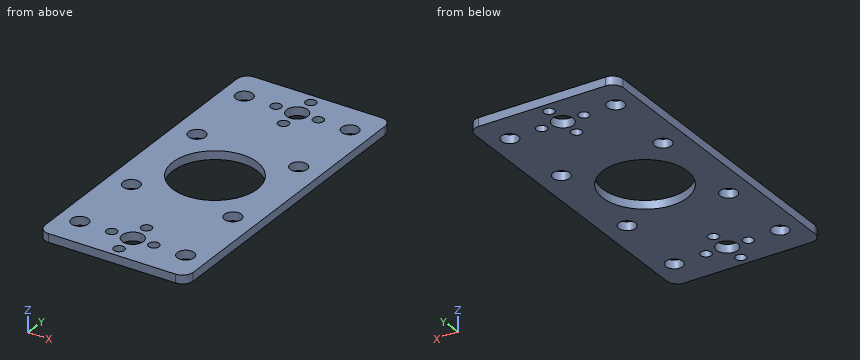
from build123d import *

# Parameters (mm, degrees)
SKETCH1_W               = 70
SKETCH1_H               = 150
SKETCH1_R               = 20
SKETCH1_R_2             = 4
BASE_FLANGE1_DEPTH      = 4
FILLET1_R               = 5
CUT_EXTRUDE1_DEPTH      = 84.903688401
CUT_EXTRUDE1_DEPTH_BACK = 4
SKETCH2_R               = 5
SKETCH3_R               = 2.5
CUT_EXTRUDE2_DEPTH      = 4


# Sheet-metal steps are written as plain solids
with BuildPart() as part:
    # Sketch1 → Base-Flange1 (new body)
    with BuildSketch(Plane.XY):
        with Locations((1.028252341, 0.668976209)):
            Rectangle(SKETCH1_W, SKETCH1_H)
        with Locations((1.028252341, 0.668976209)):
            Circle(SKETCH1_R, mode=Mode.SUBTRACT)
        with Locations((-22.971747659, 24.668976209)):
            Circle(SKETCH1_R_2, mode=Mode.SUBTRACT)
        with Locations((25.028252341, 24.668976209)):
            Circle(SKETCH1_R_2, mode=Mode.SUBTRACT)
        with Locations((25.028252341, -23.331023791)):
            Circle(SKETCH1_R_2, mode=Mode.SUBTRACT)
        with Locations((-22.971747659, -23.331023791)):
            Circle(SKETCH1_R_2, mode=Mode.SUBTRACT)
        with Locations((26.028252341, 60.668976209)):
            Circle(SKETCH1_R_2, mode=Mode.SUBTRACT)
        with Locations((-23.971747659, 60.668976209)):
            Circle(SKETCH1_R_2, mode=Mode.SUBTRACT)
        with Locations((26.028252341, -59.331023791)):
            Circle(SKETCH1_R_2, mode=Mode.SUBTRACT)
        with Locations((-23.971747659, -59.331023791)):
            Circle(SKETCH1_R_2, mode=Mode.SUBTRACT)
    extrude(amount=-BASE_FLANGE1_DEPTH)

    # Fillet1
    fillet1_edges = [part.edges().sort_by_distance(p)[0] for p in [
        (-33.971747659, 75.668976209, -2),
        (36.028252341, 75.668976209, -2),
        (36.028252341, -74.331023791, -2),
        (-33.971747659, -74.331023791, -2),
    ]]
    fillet(fillet1_edges, radius=FILLET1_R)

    # Sketch2 → Cut-Extrude1 (cut, two sides: drawn at the far end of the back side and taken through both)
    with BuildSketch(Plane.XY.offset(-CUT_EXTRUDE1_DEPTH_BACK)):
        with Locations((1.028252341, 60.668976209)):
            Circle(SKETCH2_R)
        with Locations((1.028252341, -59.331023791)):
            Circle(SKETCH2_R)
    extrude(amount=CUT_EXTRUDE1_DEPTH + CUT_EXTRUDE1_DEPTH_BACK, mode=Mode.SUBTRACT)

    # Sketch3 → Cut-Extrude2 (cut)
    with BuildSketch(Plane.XY):
        with Locations((1.028252341, 70.668976209)):
            Circle(SKETCH3_R)
        with Locations((11.028252341, 60.668976209)):
            Circle(SKETCH3_R)
        with Locations((1.028252341, 50.668976209)):
            Circle(SKETCH3_R)
        with Locations((-8.971747659, 60.668976209)):
            Circle(SKETCH3_R)
        with Locations((-8.971747659, -59.331023791)):
            Circle(SKETCH3_R)
        with Locations((1.028252341, -49.331023791)):
            Circle(SKETCH3_R)
        with Locations((11.028252341, -59.331023791)):
            Circle(SKETCH3_R)
        with Locations((1.028252341, -69.331023791)):
            Circle(SKETCH3_R)
    extrude(amount=-CUT_EXTRUDE2_DEPTH, mode=Mode.SUBTRACT)


solid = part.part
Geometry check sheet. Reference: the model listing, model coordinates, mm. Coordinates: 2 decimals unless noted, no trailing zeros. Write each loop counter-clockwise with the first axis right and the second up, starting at its lowest first coordinate (ties: lowest second). Pieces come first, ordered by that corner, then holes. Notation, with made-up numbers: (16, -2.75) -> (54, -2.75) arc R21 cw to (54, 15.25) -> close; hole circle Ø5 at (57.25, 19). An arc over 180 degrees is marked (long way). One line per question, with ' | ' between items.
1. Cross-section at B-B on y = -5. Record the cut outline in (x, z), and give its area (3 significant figures).
Answers:
outline: (-33.97, -4) -> (-18.15, -4) -> (-18.15, 0) -> (-33.97, 0) -> close; (20.21, -4) -> (36.03, -4) -> (36.03, 0) -> (20.21, 0) -> close | area: 127 mm²
2. Cross-section at D-D on x = -15.5. Record the cut outline in (y, z), and give its area (3 significant figures).
Answers:
outline: (-74.33, -4) -> (-10.59, -4) -> (-10.59, 0) -> (-74.33, 0) -> close; (11.93, -4) -> (75.67, -4) -> (75.67, 0) -> (11.93, 0) -> close | area: 510 mm²
3. Cross-section at A-A on x = 1. State how many separate pieces and enclosed holes the cut face has, and give its area (3 significant figures).
Answers:
separate pieces: 8 | enclosed holes: 0 | area: 280 mm²
4. Depth check by flat-ended pin: pin 1 Ø5 at (x, y) = (-23.97, 60.67) entering from -Z; pin 2 Ø16 at (x, y) = (1.03, 60.67) entering from -Z. Enter the tip coordinate at first touch or a pass-through.
Answers:
pin 1: passes through | pin 2: stops at z = -4
5. Thickness scan on probe 1 along Y at (x, z) = (9.5, -2.45); probe 2 along Y at (x, z) = (13, -0.95); probe 3 along Y at (x, z) = (-21.5, -3.2). Record the ranges inside material, lowest first. Write a range as from..to.
Answers:
probe 1: y = -74.33..-61.31, -57.35..-17.45, 18.79..58.69, 62.65..75.67 | probe 2: y = -74.33..-60.87, -57.79..-15.35, 16.69..59.13, 62.21..75.67 | probe 3: y = -74.33..-62.48, -56.19..-27.05, -19.61..20.95, 28.39..57.52, 63.81..75.67
